Part print with two shaded views. Sizes in mm from the minimum x, y, z corner. A direction names the side the tool comes from. Give positions to 0.01 mm unless a question says otherwise; leave off trailing zeros. Order: outer loops, then holes, each group sorted by start corner. A loop starts at its lowest first (then second) coordinate and runs counter-clockwise, first axis right, second up. Notation, with made-up numbers: M 8.25,68 L 43.25,68 A18 cw 43.25,80 Z; hole C 6,55.25 d9. An arc over 180 degrees is marked long. Return JSON: item names as keys, results as strings. Group by question number.
1. Wall check: probe 1 along Z at (x, y) = (40, 47); probe 2 along Y at (x, z) = (40, 8.75); probe 3 along X at (y, z) = (42.5, 8). Give the ranges that are in metal, low to high. Write a range as [from, to].
2. 3-axis set-ups, long thin cutter, end or side, ignore diameter. For the marked faces 4 and 5: which of +Z, -Z, +X, -X, +Y, -Y reach the whole face in a straight line?
3. Pin check, flat tips, straight feed: pin 1 (24 mm diameter, centred on x = 24, y = 56, fed in from +Z); pin 2 (12 mm diameter, centred on y = 39, z = 15.5, fed in from +X); pin 3 (3 mm diameter, centred on x = 36, z = 13, fed in from -Y); pin 4 (4.5 mm diameter, centred on x = 40, z = 15, fed in from -Y). Stop position of each tip, or through.
4. Two-plate mould, pull along Y, no slides. Class the marked faces 1, 2 and 3: released by +Y, released by -Y, zero draft, split by the parting line, or undercut.
5. Slice it at C-C on z = 4.75. List the corners of the cut face in (x, y).
6. Slice it at B-B on y = 40. List the corners of the cut face in (x, z).
7. Slice it at A-A on x = 40. List the corners of the cut face in (y, z), then the cut area to 4 significant figures.
8. Slice it at D-D on x = 32. List the corners of the cut face in (y, z), then the cut area to 3 significant figures.
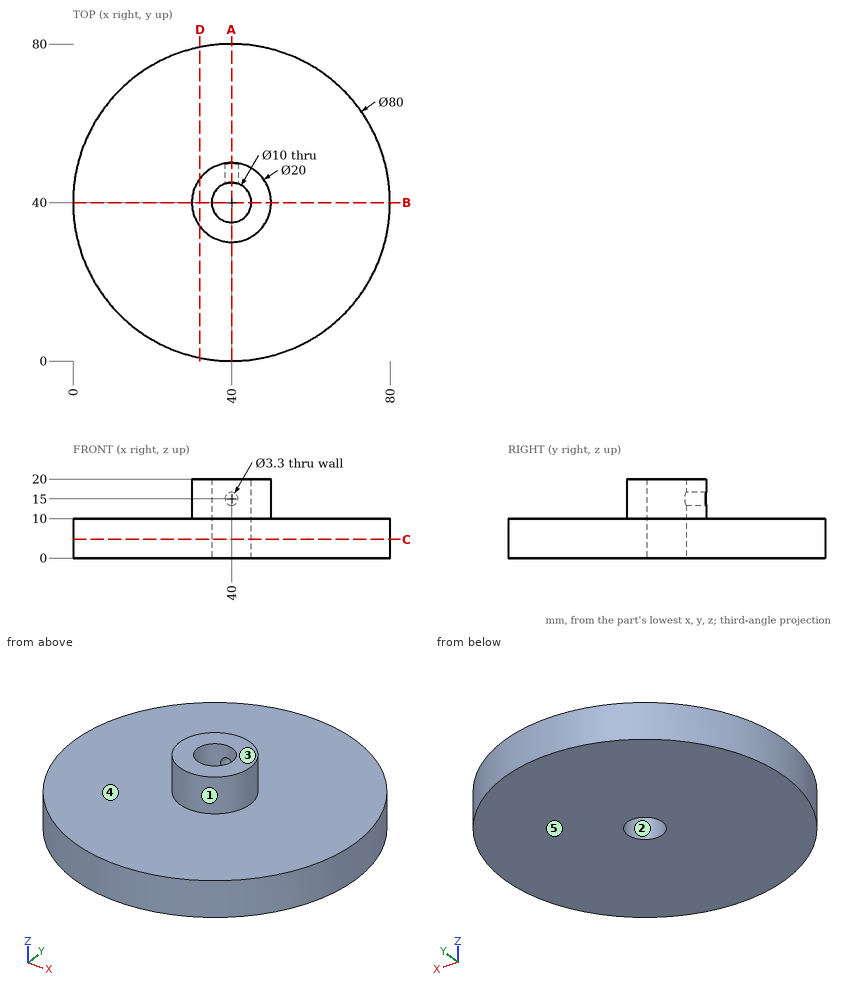
Result:
{
 "1": {"probe 1": "z = [0, 13.35], [16.65, 20]", "probe 2": "y = [0, 35], [45, 80]", "probe 3": "x = [0.08, 35.67], [44.33, 79.92]"},
 "2": {"face 4": "+Z", "face 5": "-Z, +X, -X, +Y, -Y"},
 "3": {"pin 1": "stops at z = 10", "pin 2": "stops at x = 80", "pin 3": "stops at y = 30.32", "pin 4": "stops at y = 30"},
 "4": {"face 1": "split by the parting line", "face 2": "undercut", "face 3": "zero draft"},
 "5": {"outline": "C 40,40 d80; hole C 40,40 d10"},
 "6": {"outline": "M 0,0 L 35,0 L 35,20 L 30,20 L 30,10 L 0,10 Z; M 45,0 L 80,0 L 80,10 L 50,10 L 50,20 L 45,20 Z"},
 "7": {"outline": "M 0,0 L 35,0 L 35,20 L 30,20 L 30,10 L 0,10 Z; M 45,0 L 80,0 L 80,10 L 50,10 L 50,13.35 L 45,13.35 Z; M 45,16.65 L 50,16.65 L 50,20 L 45,20 Z", "area": "783.5 mm2"},
 "8": {"outline": "M 0.81,0 L 79.19,0 L 79.19,10 L 46,10 L 46,20 L 34,20 L 34,10 L 0.81,10 Z", "area": "904 mm2"}
}
